from build123d import *

# Parameters (mm, degrees)
SKETCH1_W           = 92
SKETCH1_H           = 92
BOSS_EXTRUDE1_DEPTH = 25.5
SKETCH2_R           = 2
CUT_EXTRUDE1_DEPTH  = 26.5
FILLET1_R           = 4
SKETCH3_R           = 45
CUT_EXTRUDE2_DEPTH  = 2
SKETCH4_R           = 45
CUT_EXTRUDE3_DEPTH  = 2


with BuildPart() as part:
    # Sketch1 → Boss-Extrude1 (new body)
    with BuildSketch(Plane.XY):
        Rectangle(SKETCH1_W, SKETCH1_H)
    extrude(amount=BOSS_EXTRUDE1_DEPTH)

    # Sketch2 → Cut-Extrude1 (cut, through all)
    with BuildSketch(Plane.XY.offset(25.5)):
        with Locations((-41.25, 41.25)):
            Circle(SKETCH2_R)
        with Locations((41.25, 41.25)):
            Circle(SKETCH2_R)
        with Locations((41.25, -41.25)):
            Circle(SKETCH2_R)
        with Locations((-41.25, -41.25)):
            Circle(SKETCH2_R)
    extrude(amount=-CUT_EXTRUDE1_DEPTH, mode=Mode.SUBTRACT)

    # Fillet1
    fillet1_edges = [part.edges().sort_by_distance(p)[0] for p in [
        (46, -46, 12.75),
        (-46, -46, 12.75),
        (-46, 46, 12.75),
        (46, 46, 12.75),
    ]]
    fillet(fillet1_edges, radius=FILLET1_R)

    # Sketch3 → Cut-Extrude2 (cut)
    with BuildSketch(Plane.XY.offset(25.5)):
        Circle(SKETCH3_R)
    extrude(amount=-CUT_EXTRUDE2_DEPTH, mode=Mode.SUBTRACT)

    # Sketch4 → Cut-Extrude3 (cut)
    with BuildSketch(Plane(origin=(0, 0, 0), x_dir=(-1, 0, 0), z_dir=(0, 0, -1))):
        Circle(SKETCH4_R)
    extrude(amount=-CUT_EXTRUDE3_DEPTH, mode=Mode.SUBTRACT)


solid = part.part
Design review of the part built by this model. Coordinates are the model's own, in mm. A direction names the side the tool comes from. Round coordinates to 2 decimals unless told otherwise and drop trailing zeros. Order: outer loops, then holes, each group sorted by start corner. A loop starts at its lowest first (then second) coordinate and runs counter-clockwise, first axis right, second up. Notation, with made-up numbers: M -5.75,23 L 40.25,23 A10 cw 40.25,37 Z; hole C 29,-6.75 d9. An arc over 180 degrees is marked long. Answer as CSV lines item,"result". Start each with the question number.
1) Add section B-B (x = -29.5). Give the boundary of the cut face in (y, z).
2) Add section A-A (y = 0). Give the boundary of the cut face in (x, z).
3) For pin 1 Ø5 at (x, y) = (41.25, 41.25) entering from +Z; pin 2 Ø6 at (x, y) = (-33, 14.5) entering from +Z; pin 3 Ø1 at (x, y) = (-18, 11) entering from -Z, all flat-tipped, find the tip position at first contact; note any pin that passes through.
4) The part is to be moulded in two halves that separate along X. For faces 1 (the face through (-41.7, -43.2, 12.9)), 2 (the face through (44.797, 44.859, 12.928)), 3 (the face through (-1, 46, 13)), say which applies: +X half, -X half, draft (parallel to the pull), parting line (faces both ways), or undercut.
5) Wall thickness on line 1 along Y through (x, z) = (-41.25, 16.5); line 2 along Y through (x, z) = (0, 0.9); line 3 along X through (y, z) = (40, 24.75): over which ranges is each line inside the solid? List them lowest first. Write a range as [from, to].
6) Tool access review of faces 4 (the face through (-20.765, -39.923, 0.986)), 5 (the face through (20.765, -39.923, 24.514)), 6 (the face through (-46, -1, 13)): name each direction out of +Z, -Z, +X, -X, +Y, -Y from which nothing blocks a thin tool from reaching the whole face with its end or side.
Resolved:
1,outline,"M -46,0 L -33.98,0 L -33.98,2 L 33.98,2 L 33.98,0 L 46,0 L 46,25.5 L 33.98,25.5 L 33.98,23.5 L -33.98,23.5 L -33.98,25.5 L -46,25.5 Z"
2,outline,"M -46,0 L -45,0 L -45,2 L 45,2 L 45,0 L 46,0 L 46,25.5 L 45,25.5 L 45,23.5 L -45,23.5 L -45,25.5 L -46,25.5 Z"
3,pin 1,"z = 25.5"
3,pin 2,"z = 23.5"
3,pin 3,"z = 2"
4,face 1,"undercut"
4,face 2,"+X half"
4,face 3,"draft"
5,line 1,"[-46, -43.25], [-39.25, 39.25], [43.25, 46]"
5,line 2,"[-46, -45], [45, 46]"
5,line 3,"[-46, -42.81], [-39.69, -20.62], [20.62, 39.69], [42.81, 46]"
6,face 4,"-Z"
6,face 5,"+Z"
6,face 6,"+Z, -Z, -X, +Y, -Y"
